```python
from build123d import *

# Parameters (mm, degrees)
F1_DEPTH = 10
F2_DEPTH = 6
F3_W     = 4
F3_H     = 32
F4_DEPTH = 16.001


with BuildPart() as f1:
    # F0 (on Top) → F1 (new body)
    with BuildSketch(Plane.XY):
        with BuildLine():
            ThreePointArc((-2.25, -6.25), (0, -8.5), (2.25, -6.25))
            ThreePointArc((2.25, -6.25), (0, -4), (-2.25, -6.25))
        make_face()
    extrude(amount=F1_DEPTH)

    # F0 (on Top) → F2 (join)
    with BuildSketch(Plane.XY):
        with BuildLine():
            ThreePointArc((-2.25, -6.25), (0, -8.5), (2.25, -6.25))
            ThreePointArc((2.25, -6.25), (0, -4), (-2.25, -6.25))
        make_face()
        with BuildLine():
            ThreePointArc((-2.25, -6.25), (0, -4), (2.25, -6.25))
            Line((2.25, -6.25), (2.25, 0))
            Line((2.25, 0), (-2.25, 0))
            Line((-2.25, 0), (-2.25, -6.25))
        make_face()
        with BuildLine():
            Line((2.25, -32), (2.25, -6.25))
            ThreePointArc((2.25, -6.25), (0, -8.5), (-2.25, -6.25))
            Line((-2.25, -6.25), (-2.25, -32))
            Line((-2.25, -32), (2.25, -32))
        make_face()
    extrude(amount=-F2_DEPTH)

    # F3 (on face) → F4 (intersect, through all)
    with BuildSketch(Plane(origin=(0, 0, -6), x_dir=(1, 0, 0), z_dir=(0, 0, -1))):
        with Locations((0, 16)):
            Rectangle(F3_W, F3_H)
    extrude(amount=-F4_DEPTH, mode=Mode.INTERSECT)


solid = f1.part
```
Could you check a few things on this model? Use its own coordinates, in mm. A direction names the side the tool comes from. Round coordinates to 2 decimals unless told otherwise and drop trailing zeros. Loops run counter-clockwise (first coordinate to the right, second up) from the corner with the lowest first, then second, coordinate; pieces in that order, holes last.
Q1. For P1, Ø2, axis at x = -1.5, y = -13.5, coming from the +Z side; P2, Ø1.5, axis at y = -11.5, z = 1, coming from the -X side, each with a flat end and sliding along its axis, tell me the tip position at first contact or that it passes through.
Q2. I want a section at C-C (z = 7.25). Write out the boundary of the cut face in (x, y).
Q3. I want a section at D-D (x = 0.8). Write out the boundary of the cut face in (y, z), and give its area (3 significant figures).
Q4. I want a section at B-B (y = -27). Write out the boundary of the cut face in (x, z).
Q5. Please list where these lines run through material, in increasing order: L1, parallel to Z at x = -0.65, y = -30; L2, parallel to Y at x = -0.1, z = 5; L3, parallel to Y at x = -0.65, z = 4.5.
Q6. On a 3-axis mill with a long thin cutter (end or side, diameter ignored), from which of +Z, -Z, +X, -X, +Y, -Y can I reach the whole of each face in a straight line? I mean faces 1 (the flat face through (0, -32, -3)), 2 (the cylindrical face through (0, -4, 5)), 3 (the cylindrical face through (0, -8.5, 4.9)). Say none if no direction works.
Q7. I want a section at A-A (x = -0.6). Write out the boundary of the cut face in (y, z).
Answer below:
1. P1: stops at z = 0
1. P2: passes through
2. outline: (-2, -7.28) arc R2.25 ccw to (2, -7.28) - (2, -5.22) arc R2.25 ccw to (-2, -5.22) - close
3. outline: (-32, -6) - (0, -6) - (0, 0) - (-4.15, 0) - (-4.15, 10) - (-8.35, 10) - (-8.35, 0) - (-32, 0) - close
3. area: 234 mm2
4. outline: (-2, -6) - (2, -6) - (2, 0) - (-2, 0) - close
5. L1: z = -6 to 0
5. L2: y = -8.5 to -4
5. L3: y = -8.4 to -4.1
6. face 1: +Z, -Z, +X, -X, -Y
6. face 2: +Z, +Y
6. face 3: +Z, -Y
7. outline: (-32, -6) - (0, -6) - (0, 0) - (-4.08, 0) - (-4.08, 10) - (-8.42, 10) - (-8.42, 0) - (-32, 0) - close
